```python
from build123d import *

# Parameters (mm, degrees)
BOSS_EXTRUDE1_DEPTH = 3.175
FILLET1_R           = 2.38125
SKETCH2_R           = 2.4511
SKETCH2_R_2         = 9.652
SKETCH2_R_3         = 7.62
SKETCH2_R_4         = 9.1186
CUT_EXTRUDE1_DEPTH  = 292.413808153


with BuildPart() as part:
    # Sketch1 → Boss-Extrude1 (new body)
    with BuildSketch(Plane(origin=(0, 0, 0), x_dir=(1, 0, 0), z_dir=(0, 1, 0))):
        Polygon((-158.623, 114.3), (-217.719823012, 61.309848699), (-115.230823012, -52.990151301), (-56.134, 0), (-56.134, -79.375), (56.134, -79.375), (56.134, 0), (115.230823012, -52.990151301), (217.719823012, 61.309848699), (158.623, 114.3), (158.623, 193.675), (-158.623, 193.675), align=None)
    extrude(amount=BOSS_EXTRUDE1_DEPTH)

    # Fillet1
    fillet1_edges = [part.edges().sort_by_distance(p)[0] for p in [
        (-56.134, 1.5875, 0),
        (-158.623, 1.5875, -114.3),
        (158.623, 1.5875, -114.3),
        (56.134, 1.5875, 0),
    ]]
    fillet(fillet1_edges, radius=FILLET1_R)

    # Sketch2 → Cut-Extrude1 (cut, through all)
    with BuildSketch(Plane(origin=(0, 3.175, 0), x_dir=(1, 0, 0), z_dir=(0, 1, 0))):
        with Locations(Location((52.705, 147.8915, 0), (0, 0, 270))):
            Circle(SKETCH2_R)
        with Locations(Location((10.795, 147.8915, 0), (0, 0, 270))):
            Circle(SKETCH2_R)
        with Locations(Location((-10.795, 147.8915, 0), (0, 0, 270))):
            Circle(SKETCH2_R)
        with Locations(Location((-52.705, 147.8915, 0), (0, 0, 270))):
            Circle(SKETCH2_R)
        with Locations(Location((-109.855, 147.8915, 0), (0, 0, 270))):
            Circle(SKETCH2_R_2)
        with Locations(Location((-78.105, 147.8915, 0), (0, 0, 270))):
            Circle(SKETCH2_R_3)
        with Locations(Location((78.105, 147.8915, 0), (0, 0, 270))):
            Circle(SKETCH2_R_3)
        with Locations(Location((109.855, 147.8915, 0), (0, 0, 270))):
            Circle(SKETCH2_R_4)
        with BuildLine():
            Line((17.7165, 157.1498), (17.7165, 138.6332))
            ThreePointArc((17.7165, 138.6332), (19.115123698, 135.256623698), (22.4917, 133.858))
            Line((22.4917, 133.858), (41.0083, 133.858))
            ThreePointArc((41.0083, 133.858), (44.384876302, 135.256623698), (45.7835, 138.6332))
            Line((45.7835, 138.6332), (45.7835, 157.1498))
            ThreePointArc((45.7835, 157.1498), (44.384876302, 160.526376302), (41.0083, 161.925))
            Line((41.0083, 161.925), (22.4917, 161.925))
            ThreePointArc((22.4917, 161.925), (19.115123698, 160.526376302), (17.7165, 157.1498))
        make_face()
        with BuildLine():
            Line((-45.7835, 157.1498), (-45.7835, 138.6332))
            ThreePointArc((-45.7835, 138.6332), (-44.384876302, 135.256623698), (-41.0083, 133.858))
            Line((-41.0083, 133.858), (-22.4917, 133.858))
            ThreePointArc((-22.4917, 133.858), (-19.115123698, 135.256623698), (-17.7165, 138.6332))
            Line((-17.7165, 138.6332), (-17.7165, 157.1498))
            ThreePointArc((-17.7165, 157.1498), (-19.115123698, 160.526376302), (-22.4917, 161.925))
            Line((-22.4917, 161.925), (-41.0083, 161.925))
            ThreePointArc((-41.0083, 161.925), (-44.384876302, 160.526376302), (-45.7835, 157.1498))
        make_face()
    extrude(amount=-CUT_EXTRUDE1_DEPTH, mode=Mode.SUBTRACT)


solid = part.part
```
Geometry check sheet. Reference: the model listing, model coordinates, mm. A direction names the side the tool comes from. Give positions to 0.01 mm unless a question says otherwise; leave off trailing zeros. Write each loop counter-clockwise with the first axis right and the second up, starting at its lowest first coordinate (ties: lowest second). Pieces come first, ordered by that corner, then holes. Notation, with made-up numbers: (85.25, 65.25) -> (109.25, 65.25) arc R22 ccw to (109.25, 90.25) -> close; hole circle Ø4 at (-37.75, -18). An arc over 180 degrees is marked (long way). Use one line per item in the form item = value.
Item 1: Mould release check, pull along X, two halves, no side actions. Record for faces 1 (the flat face through (-188.159, 1.565, -87.816)), 2 (the flat face through (-3, 0, -59)), 3 (the cylindrical face through (-77.77, 1.61, -155.504)): released by +X, released by -X, zero draft, split by the parting line, or undercut.
Results list:
face_1 = released by -X
face_2 = zero draft
face_3 = undercut
Item 2: Sectioned sample at D-D on z = -48. Enter the section's corners in (x, y) (3 decimals).
Results list:
outline = (-205.785, 0) -> (205.785, 0) -> (205.785, 3.175) -> (-205.785, 3.175) -> close
Item 3: Scan lines: line 1 (Z direction, x = 37.5, y = 1.25) (3 decimals); line 2 (X direction, y = 1.5, z = 40.5); line 3 (X direction, y = 2.5, z = 7). Record each from-to range of solid material in increasing order.
Results list:
line_1 = -193.675 to -161.925, -133.858 to 79.375
line_2 = -126.43 to -101.3, -56.13 to 56.13, 101.3 to 126.43
line_3 = -156.47 to -63.94, -56.13 to 56.13, 63.94 to 156.47
Item 4: Access from +Z, -Z, +X, -X, +Y, -Y to the whole of each face (thin tool, end or side, straight path). Record for faces 4 (the flat face through (-3, 3.175, -59)), 5 (the flat face through (-88.05, 1.57, 28.62)).
Results list:
face_4 = +Z, -Z, +X, -X, +Y
face_5 = +Z, +Y, -Y
Item 5: Sectioned sample at B-B on z = -120.5. Enter the section's corners in (x, y) (3 decimals), plus the area to 3 significant figures.
Results list:
outline = (-158.623, 0) -> (158.623, 0) -> (158.623, 3.175) -> (-158.623, 3.175) -> close
area = 1,010 mm2
Item 6: Depth check by flat-ended pin: pin 1 Ø16.5 at (x, z) = (109.86, -147.89) entering from +Y; pin 2 Ø1.5 at (y, z) = (2.5, 35.5) entering from -X; pin 3 Ø4 at (x, z) = (53, -74.5) entering from -Y; pin 4 Ø1.5 at (y, z) = (2.5, -10.5) entering from -X. Enter the tip coordinate at first touch or a pass-through.
Results list:
pin_1 = through
pin_2 = -131.59
pin_3 = 0
pin_4 = -172.83
Item 7: Sectioned sample at C-C on y = 1.15. Count the separate pieces of the cut face and the enclosed holes in it, plus the area to 3 significant figures.
Results list:
separate_pieces = 1
enclosed_holes = 10
area = 80,500 mm2
Item 8: Sectioned sample at A-A on x = -29. Enter the section's corners in (y, z) (3 decimals), plus the area to 3 significant figures.
Results list:
outline = (0, -193.675) -> (3.175, -193.675) -> (3.175, -161.925) -> (0, -161.925) -> close; (0, -133.858) -> (3.175, -133.858) -> (3.175, 79.375) -> (0, 79.375) -> close
area = 778 mm2
